Build history of the part. All positions in model axes, mm. Face numbers are marked on the shaded views. A direction names the side the tool comes from. Give positions to 0.01 mm unless a question says otherwise; leave off trailing zeros. Loops run counter-clockwise (first coordinate to the right, second up) from the corner with the lowest first, then second, coordinate; pieces in that order, holes last.
1) Band-saw the part on C-C on y = 58.5. List the corners of the cut face in (x, z) (3 decimals).
2) Band-saw the part on D-D on x = 33.5. List the corners of the cut face in (y, z) (3 decimals).
3) Band-saw the part on A-A on y = 68. List the corners of the cut face in (x, z) (3 decimals).
4) 3-axis set-ups, long thin cutter, end or side, ignore diameter. For the marked faces 1 and 2: which of +Z, -Z, +X, -X, +Y, -Y reach the whole face in a straight line?
5) Flat gauge pins, fed straight in: P1, Ø8, axis at x = 38, z = 9, coming from the +Y side; P2, Ø7, axis at y = 38.5, z = 59.85, coming from the +X side (3 decimals); P3, Ø3, axis at x = 43, y = 16.5, coming from the +Z side (3 decimals). Where does each tip first touch, or does it go through?
6) Wall check: line 1 (Z direction, x = 1.4, y = 58.5); line 2 (Z direction, x = 12.5, y = 39.5) (3 decimals). Give the ranges that are in metal, low to high.
7) Band-saw the part on B-B on z = 59.85. List the corners of the cut face in (x, y) (3 decimals), then the cut area to 3 significant figures.
```python
from build123d import *

# Parameters (mm, degrees)
CROQUIS2_W              = 50.8
CROQUIS2_H              = 80
SALIENTE_EXTRUIR1_DEPTH = 3.175
CROQUIS3_W              = 3.175
CROQUIS3_H              = 80
SALIENTE_EXTRUIR2_DEPTH = 66.675
CROQUIS4_R              = 2.75
CORTAR_EXTRUIR1_DEPTH   = 47.625
CROQUIS5_R              = 3
CORTAR_EXTRUIR2_DEPTH   = 47.625


with BuildPart() as part:
    # Croquis2 → Saliente-Extruir1 (new body)
    with BuildSketch(Plane.XY):
        with Locations((25.4, 40)):
            Rectangle(CROQUIS2_W, CROQUIS2_H)
    extrude(amount=SALIENTE_EXTRUIR1_DEPTH)

    # Croquis3 → Saliente-Extruir2 (add)
    with BuildSketch(Plane.XY.offset(3.175)):
        with Locations((1.5875, 40)):
            Rectangle(CROQUIS3_W, CROQUIS3_H)
    extrude(amount=SALIENTE_EXTRUIR2_DEPTH)

    # Croquis4 → Cortar-Extruir1 (cut)
    with BuildSketch(Plane.XY.offset(3.175)):
        with Locations((13.175, 68)):
            Circle(CROQUIS4_R)
        with Locations((13.175, 12)):
            Circle(CROQUIS4_R)
        with Locations((34.175, 68)):
            Circle(CROQUIS4_R)
        with Locations((34.175, 12)):
            Circle(CROQUIS4_R)
    extrude(amount=-CORTAR_EXTRUIR1_DEPTH, mode=Mode.SUBTRACT)

    # Croquis5 → Cortar-Extruir2 (cut)
    with BuildSketch(Plane(origin=(3.175, 0, 0), x_dir=(0, 0, -1), z_dir=(1, 0, 0))):
        with Locations(Location((-59.85, 18.5, 0), (0, 0, 90))):
            Circle(CROQUIS5_R)
        with Locations(Location((-59.85, 38.5, 0), (0, 0, 90))):
            Circle(CROQUIS5_R)
        with Locations(Location((-59.85, 58.5, 0), (0, 0, 90))):
            Circle(CROQUIS5_R)
    extrude(amount=-CORTAR_EXTRUIR2_DEPTH, mode=Mode.SUBTRACT)


solid = part.part
```
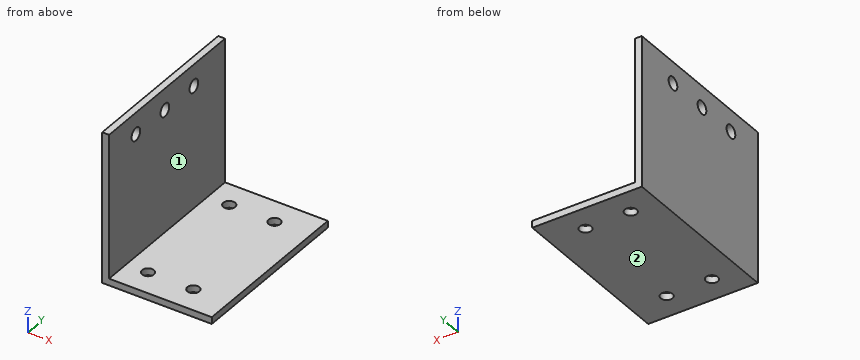
Findings below:
1. outline: (0, 0) - (50.8, 0) - (50.8, 3.175) - (3.175, 3.175) - (3.175, 56.85) - (0, 56.85) - close; (0, 62.85) - (3.175, 62.85) - (3.175, 69.85) - (0, 69.85) - close
2. outline: (0, 0) - (9.334, 0) - (9.334, 3.175) - (0, 3.175) - close; (14.666, 0) - (65.334, 0) - (65.334, 3.175) - (14.666, 3.175) - close; (70.666, 0) - (80, 0) - (80, 3.175) - (70.666, 3.175) - close
3. outline: (0, 0) - (10.425, 0) - (10.425, 3.175) - (3.175, 3.175) - (3.175, 69.85) - (0, 69.85) - close; (15.925, 0) - (31.425, 0) - (31.425, 3.175) - (15.925, 3.175) - close; (36.925, 0) - (50.8, 0) - (50.8, 3.175) - (36.925, 3.175) - close
4. face 1: +Z, +X, +Y, -Y
4. face 2: -Z, +X, -X, +Y, -Y
5. P1: passes through
5. P2: stops at x = 3.175
5. P3: stops at z = 3.175
6. line 1: z = 0 to 56.85, 62.85 to 69.85
6. line 2: z = 0 to 3.175
7. outline: (0, 0) - (3.175, 0) - (3.175, 15.5) - (0, 15.5) - close; (0, 21.5) - (3.175, 21.5) - (3.175, 35.5) - (0, 35.5) - close; (0, 41.5) - (3.175, 41.5) - (3.175, 55.5) - (0, 55.5) - close; (0, 61.5) - (3.175, 61.5) - (3.175, 80) - (0, 80) - close
7. area: 197 mm2
